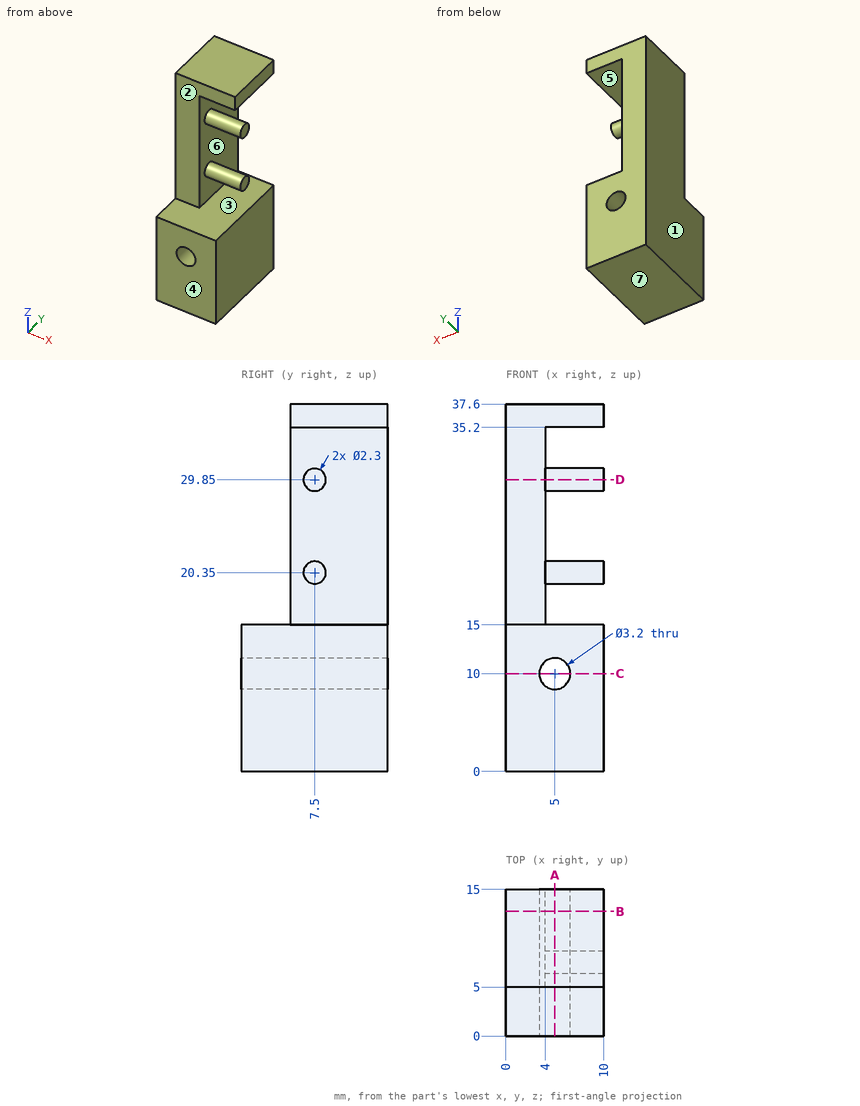
Answer from the drawing. Dimensions are ordinates in mm from the lowest x, y and z of the part. A direction names the side the tool comes from. Give positions to 0.01 mm unless a question says otherwise; leave off trailing zeros. Loops run counter-clockwise (first coordinate to the right, second up) from the corner with the lowest first, then second, coordinate; pieces in that order, holes last. Notation, with made-up numbers: (0, 27) - (20, 27) arc R28 ccw to (20, 58) - close; hole circle Ø11 at (10.25, 29.5). An arc over 180 degrees is marked (long way). Answer as a JSON object with one key per item and string values.
1. For the marked faces 1, 2 and 3, determine the directions among +Z, -Z, +X, -X, +Y, -Y from which every point of the face is accessible in a straight line to the end or side of a thin tool.
Determined:
{"face 1": "+Z, -Z, -X, +Y, -Y", "face 2": "+Z, +X, -X, -Y", "face 3": "+X, -Y"}
2. A cutting plane is placed at A-A (x = 5). Write down the section's boundary in (y, z), then the cut area to 3 significant figures.
Determined:
{"outline": "(0, 0) - (15, 0) - (15, 8.4) - (0, 8.4) - close; (0, 11.6) - (15, 11.6) - (15, 15) - (0, 15) - close; (5, 35.2) - (15, 35.2) - (15, 37.6) - (5, 37.6) - close; circle Ø2.3 at (7.5, 20.35); circle Ø2.3 at (7.5, 29.85)", "area": "209 mm²"}
3. A cutting plane is placed at D-D (z = 29.85). Write down the section's boundary in (x, y), then the cut area to 3 significant figures.
Determined:
{"outline": "(0, 5) - (4, 5) - (4, 6.35) - (10, 6.35) - (10, 8.65) - (4, 8.65) - (4, 15) - (0, 15) - close", "area": "53.8 mm²"}
4. Find the intervals of material crossed by L1, parallel to Z at x = 5, y = 10.5; L2, parallel to Z at x = 9.25, y = 14; L3, parallel to Y at x = 3.75, z = 33.5, in increasing order. Write a range as [from, to].
Determined:
{"L1": "[0, 8.4], [11.6, 15], [35.2, 37.6]", "L2": "[0, 15], [35.2, 37.6]", "L3": "[5, 15]"}
5. A cutting plane is placed at B-B (y = 12.75). Write down the section's boundary in (x, z), then the cut area to 3 significant figures.
Determined:
{"outline": "(0, 0) - (10, 0) - (10, 15) - (4, 15) - (4, 35.2) - (10, 35.2) - (10, 37.6) - (0, 37.6) - close; hole circle Ø3.2 at (5, 10)", "area": "247 mm²"}
6. A flat-ended cylindrical pin translates along its axis: pin 1 Ø5 at (y, z) = (11, 28.5) entering from +X. Find the tip coordinate at first contact, or state that the pin passes through.
Determined:
{"pin 1": "x = 4"}
7. A cutting plane is placed at C-C (z = 10). Write down the section's boundary in (x, y).
Determined:
{"outline": "(0, 0) - (3.4, 0) - (3.4, 15) - (0, 15) - close; (6.6, 0) - (10, 0) - (10, 15) - (6.6, 15) - close"}
8. For a pull along Z with two mould halves and no side action, classify the marked faces 4, 5, 6 and 7 as pulls with the +Z half, pulls with the -Z half, needs draft (parallel to the pull), parting line crosses it, or undercut.
Determined:
{"face 4": "needs draft", "face 5": "undercut", "face 6": "undercut", "face 7": "pulls with the -Z half"}
